The figure shows three views and two pictorial views of one solid part (mm, origin at its lowest corner). Answer the questions. A direction names the side the tool comes from. Give positions to 0.01 mm unless a question says otherwise; leave off trailing zeros. Write each loop counter-clockwise with the first axis right and the second up, starting at its lowest first coordinate (ties: lowest second). Pieces come first, ordered by that corner, then holes. Notation, with made-up numbers: (43, 20) - (65, 20) arc R17 ccw to (65, 27) - close; hole circle Ø3 at (68, 53). An arc over 180 degrees is marked (long way). Answer as CSV lines item,"result". Start each with the question number.
(1) Straight lines are drawn through the part: probe 1 along Y at (x, z) = (27, 72); probe 2 along Z at (x, y) = (63, 86); probe 3 along Z at (x, y) = (109.5, 18.5). For each, find the intervals that lie inside material, in ascending order.
(2) For the marked faces 1 and 2, determine the directions among +Z, -Z, +X, -X, +Y, -Y from which every point of the face is accessible in a straight line to the end or side of a thin tool.
(3) Each of these flat-tipped pins is pushed along its axis until it touches: pin 1 Ø1.5 at (x, y) = (72.5, 47.5) entering from -Z; pin 2 Ø1 at (x, z) = (78, 114) entering from +Y. Where does it stop, or does it pass through?
(4) Find section C-C (y = 104.5). Write down the section's boundary in (x, z).
(5) Find section A-A (x = 39.5). Write down the section's boundary in (y, z).
(6) Find section B-B (z = 101.5). Write down the section's boundary in (x, y), then the cut area to 3 significant figures.
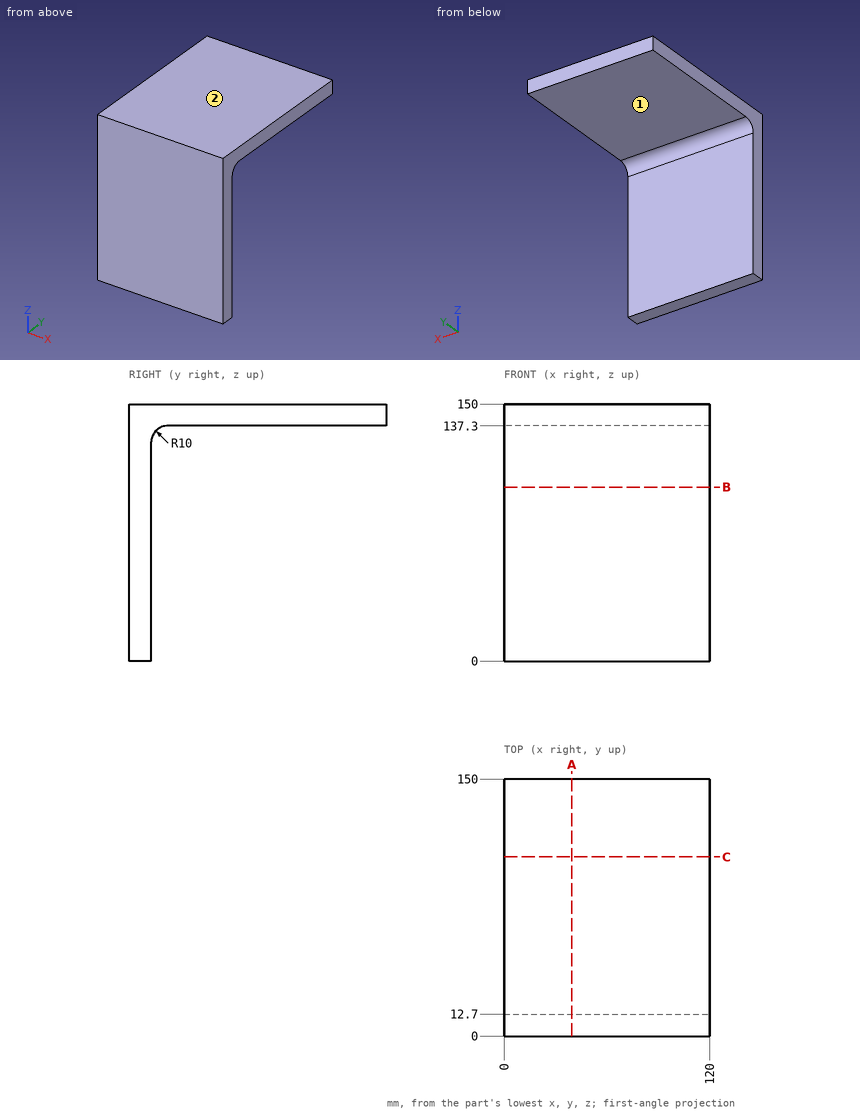
Result set:
1,probe 1,"0 to 12.7"
1,probe 2,"137.3 to 150"
1,probe 3,"136.38 to 150"
2,face 1,"-Z, +X, -X, +Y"
2,face 2,"+Z, +X, -X, +Y, -Y"
3,pin 1,"z = 137.3"
3,pin 2,"y = 12.7"
4,outline,"(0, 137.3) - (120, 137.3) - (120, 150) - (0, 150) - close"
5,outline,"(0, 0) - (12.7, 0) - (12.7, 127.3) arc R10 cw to (22.7, 137.3) - (150, 137.3) - (150, 150) - (0, 150) - close"
6,outline,"(0, 0) - (120, 0) - (120, 12.7) - (0, 12.7) - close"
6,area,"1,520 mm^2"
